```python
from build123d import *

# Parameters (mm, degrees)
F0_R     = 70
F0_W     = 10
F0_H     = 43.5
F0_W_2   = 43.5
F0_H_2   = 10
F0_R_2   = 4
F1_DEPTH = 5


with BuildPart() as f1:
    # F0 (on Top) → F1 (new body)
    with BuildSketch(Plane.XY):
        Circle(F0_R)
        with BuildLine():
            ThreePointArc((-50.419256, -41.023148), (-50.834826, -39.398712), (-49.867894, -38.028846))
            Line((-49.867894, -38.028846), (-28.320508, -25.588457))
            ThreePointArc((-28.320508, -25.588457), (-25.906295, -25.906295), (-25.588457, -28.320508))
            Line((-25.588457, -28.320508), (-38.028846, -49.867894))
            ThreePointArc((-38.028846, -49.867894), (-39.398712, -50.834826), (-41.023148, -50.419256))
            ThreePointArc((-41.023148, -50.419256), (-45.961941, -45.961941), (-50.419256, -41.023148))
        make_face(mode=Mode.SUBTRACT)
        Polygon((-6.669873, -21.552559), (-28.419873, -59.224664), (-37.080127, -54.224664), (-15.330127, -16.552559), align=None, mode=Mode.SUBTRACT)
        with BuildLine():
            ThreePointArc((-23.152782, -60.736716), (-24.324895, -59.537699), (-24.17244, -57.867894))
            Line((-24.17244, -57.867894), (-11.732051, -36.320508))
            ThreePointArc((-11.732051, -36.320508), (-9.482362, -35.388656), (-8, -37.320508))
            Line((-8, -37.320508), (-8, -62.201286))
            ThreePointArc((-8, -62.201286), (-8.702873, -63.723607), (-10.31746, -64.17593))
            ThreePointArc((-10.31746, -64.17593), (-16.823238, -62.785179), (-23.152782, -60.736716))
        make_face(mode=Mode.SUBTRACT)
        Polygon((-16.552559, -15.330127), (-54.224664, -37.080127), (-59.224664, -28.419873), (-21.552559, -6.669873), align=None, mode=Mode.SUBTRACT)
        with BuildLine():
            ThreePointArc((-64.17593, -10.31746), (-63.723607, -8.702873), (-62.201286, -8))
            Line((-62.201286, -8), (-37.320508, -8))
            ThreePointArc((-37.320508, -8), (-35.388656, -9.482362), (-36.320508, -11.732051))
            Line((-36.320508, -11.732051), (-57.867894, -24.17244))
            ThreePointArc((-57.867894, -24.17244), (-59.537699, -24.324895), (-60.736716, -23.152782))
            ThreePointArc((-60.736716, -23.152782), (-62.785179, -16.823238), (-64.17593, -10.31746))
        make_face(mode=Mode.SUBTRACT)
        with BuildLine():
            ThreePointArc((10.31746, -64.17593), (8.702873, -63.723607), (8, -62.201286))
            Line((8, -62.201286), (8, -37.320508))
            ThreePointArc((8, -37.320508), (9.482362, -35.388656), (11.732051, -36.320508))
            Line((11.732051, -36.320508), (24.17244, -57.867894))
            ThreePointArc((24.17244, -57.867894), (24.324895, -59.537699), (23.152782, -60.736716))
            ThreePointArc((23.152782, -60.736716), (16.823238, -62.785179), (10.31746, -64.17593))
        make_face(mode=Mode.SUBTRACT)
        with Locations((0, -43.75)):
            Rectangle(F0_W, F0_H, mode=Mode.SUBTRACT)
        Polygon((15.330127, -16.552559), (37.080127, -54.224664), (28.419873, -59.224664), (6.669873, -21.552559), align=None, mode=Mode.SUBTRACT)
        with BuildLine():
            ThreePointArc((41.023148, -50.419256), (39.398712, -50.834826), (38.028846, -49.867894))
            Line((38.028846, -49.867894), (25.588457, -28.320508))
            ThreePointArc((25.588457, -28.320508), (25.906295, -25.906295), (28.320508, -25.588457))
            Line((28.320508, -25.588457), (49.867894, -38.028846))
            ThreePointArc((49.867894, -38.028846), (50.834826, -39.398712), (50.419256, -41.023148))
            ThreePointArc((50.419256, -41.023148), (45.961941, -45.961941), (41.023148, -50.419256))
        make_face(mode=Mode.SUBTRACT)
        Polygon((21.552559, -6.669873), (59.224664, -28.419873), (54.224664, -37.080127), (16.552559, -15.330127), align=None, mode=Mode.SUBTRACT)
        with BuildLine():
            ThreePointArc((60.736716, -23.152782), (59.537699, -24.324895), (57.867894, -24.17244))
            Line((57.867894, -24.17244), (36.320508, -11.732051))
            ThreePointArc((36.320508, -11.732051), (35.388656, -9.482362), (37.320508, -8))
            Line((37.320508, -8), (62.201286, -8))
            ThreePointArc((62.201286, -8), (63.723607, -8.702873), (64.17593, -10.31746))
            ThreePointArc((64.17593, -10.31746), (62.785179, -16.823238), (60.736716, -23.152782))
        make_face(mode=Mode.SUBTRACT)
        with Locations((-43.75, 0)):
            Rectangle(F0_W_2, F0_H_2, mode=Mode.SUBTRACT)
        with BuildLine():
            ThreePointArc((-60.736716, 23.152782), (-59.537699, 24.324895), (-57.867894, 24.17244))
            Line((-57.867894, 24.17244), (-36.320508, 11.732051))
            ThreePointArc((-36.320508, 11.732051), (-35.388656, 9.482362), (-37.320508, 8))
            Line((-37.320508, 8), (-62.201286, 8))
            ThreePointArc((-62.201286, 8), (-63.723607, 8.702873), (-64.17593, 10.31746))
            ThreePointArc((-64.17593, 10.31746), (-62.785179, 16.823238), (-60.736716, 23.152782))
        make_face(mode=Mode.SUBTRACT)
        Polygon((-21.552559, 6.669873), (-59.224664, 28.419873), (-54.224664, 37.080127), (-16.552559, 15.330127), align=None, mode=Mode.SUBTRACT)
        with BuildLine():
            ThreePointArc((-41.023148, 50.419256), (-39.398712, 50.834826), (-38.028846, 49.867894))
            Line((-38.028846, 49.867894), (-25.588457, 28.320508))
            ThreePointArc((-25.588457, 28.320508), (-25.906295, 25.906295), (-28.320508, 25.588457))
            Line((-28.320508, 25.588457), (-49.867894, 38.028846))
            ThreePointArc((-49.867894, 38.028846), (-50.834826, 39.398712), (-50.419256, 41.023148))
            ThreePointArc((-50.419256, 41.023148), (-45.961941, 45.961941), (-41.023148, 50.419256))
        make_face(mode=Mode.SUBTRACT)
        Polygon((-15.330127, 16.552559), (-37.080127, 54.224664), (-28.419873, 59.224664), (-6.669873, 21.552559), align=None, mode=Mode.SUBTRACT)
        with BuildLine():
            Line((-11.732051, 36.320508), (-24.17244, 57.867894))
            ThreePointArc((-24.17244, 57.867894), (-24.324895, 59.537699), (-23.152782, 60.736716))
            ThreePointArc((-23.152782, 60.736716), (-16.823238, 62.785179), (-10.31746, 64.17593))
            ThreePointArc((-10.31746, 64.17593), (-8.702873, 63.723607), (-8, 62.201286))
            Line((-8, 62.201286), (-8, 37.320508))
            ThreePointArc((-8, 37.320508), (-9.482362, 35.388656), (-11.732051, 36.320508))
        make_face(mode=Mode.SUBTRACT)
        Circle(F0_R_2, mode=Mode.SUBTRACT)
        with Locations((43.75, 0)):
            Rectangle(F0_W_2, F0_H_2, mode=Mode.SUBTRACT)
        with BuildLine():
            ThreePointArc((64.17593, 10.31746), (63.723607, 8.702873), (62.201286, 8))
            Line((62.201286, 8), (37.320508, 8))
            ThreePointArc((37.320508, 8), (35.388656, 9.482362), (36.320508, 11.732051))
            Line((36.320508, 11.732051), (57.867894, 24.17244))
            ThreePointArc((57.867894, 24.17244), (59.537699, 24.324895), (60.736716, 23.152782))
            ThreePointArc((60.736716, 23.152782), (62.785179, 16.823238), (64.17593, 10.31746))
        make_face(mode=Mode.SUBTRACT)
        Polygon((16.552559, 15.330127), (54.224664, 37.080127), (59.224664, 28.419873), (21.552559, 6.669873), align=None, mode=Mode.SUBTRACT)
        with Locations((0, 43.75)):
            Rectangle(F0_W, F0_H, mode=Mode.SUBTRACT)
        with BuildLine():
            Line((8, 37.320508), (8, 62.201286))
            ThreePointArc((8, 62.201286), (8.702873, 63.723607), (10.31746, 64.17593))
            ThreePointArc((10.31746, 64.17593), (16.823238, 62.785179), (23.152782, 60.736716))
            ThreePointArc((23.152782, 60.736716), (24.324895, 59.537699), (24.17244, 57.867894))
            Line((24.17244, 57.867894), (11.732051, 36.320508))
            ThreePointArc((11.732051, 36.320508), (9.482362, 35.388656), (8, 37.320508))
        make_face(mode=Mode.SUBTRACT)
        Polygon((6.669873, 21.552559), (28.419873, 59.224664), (37.080127, 54.224664), (15.330127, 16.552559), align=None, mode=Mode.SUBTRACT)
        with BuildLine():
            Line((25.588457, 28.320508), (38.028846, 49.867894))
            ThreePointArc((38.028846, 49.867894), (39.398712, 50.834826), (41.023148, 50.419256))
            ThreePointArc((41.023148, 50.419256), (45.961941, 45.961941), (50.419256, 41.023148))
            ThreePointArc((50.419256, 41.023148), (50.834826, 39.398712), (49.867894, 38.028846))
            Line((49.867894, 38.028846), (28.320508, 25.588457))
            ThreePointArc((28.320508, 25.588457), (25.906295, 25.906295), (25.588457, 28.320508))
        make_face(mode=Mode.SUBTRACT)
    extrude(amount=F1_DEPTH)


solid = f1.part
```
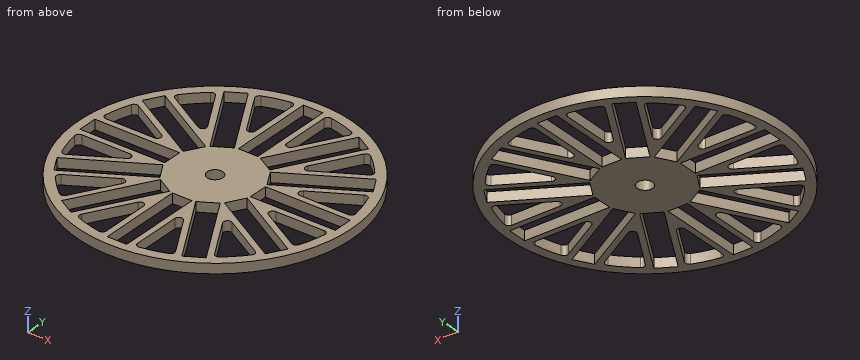
Input: part model. Units: mm. Frame: model coordinates. Give positions to 0.01 mm unless a question says otherwise; leave off trailing zeros. Order: outer loops, then holes, each group sorted by start corner. A loop starts at its lowest first (then second) coordinate and runs counter-clockwise, first axis right, second up. Notation, with made-up numbers: (55, 59.5) -> (71, 59.5) arc R24 ccw to (71, 88.5) -> close; hole circle Ø2 at (9.5, 52.25). An arc over 180 degrees is marked (long way). Write each question's results on one line, items separated by ' | '. Start each with the question number.
Item 1: Line query: line 1 (Y direction, x = 0, z = 2.4); line 2 (Y direction, x = 12.5, z = 4.05); line 3 (X direction, y = 56.5, z = 3.4). Output: solid intervals per line, ascending.
Item 2: Contact query for flat-ended pins moving along their axis: P1, Ø2, axis at y = 36.5, z = 2.5, coming from the -X side; P2, Ø3, axis at x = -10, y = -53, coming from the -Z side; P3, Ø2.5, axis at x = 47.5, z = 2, coming from the +Y side; P4, Ø1.5, axis at y = 49.5, z = 3, coming from the +X side. Output: stop coordinate, or through.
Item 3: Cut plane A-A on y = 0. Return the cut outline in (x, z), then the cut area to 3 significant figures.
Item 4: Cut plane C-C on y = -47.5. Give the number of separate pieces and of enclosed holes in the cut face, then the cut area to 3 significant figures.
Established:
1) line 1: -70 to -65.5, -22 to -4, 4 to 22, 65.5 to 70 | line 2: -68.87 to -63.79, -37.65 to -31.65, -18.19 to 18.19, 31.65 to 37.65, 63.79 to 68.87 | line 3: -41.32 to -33.14, -26.85 to -23.38, -8 to -5, 5 to 8, 23.38 to 26.85, 33.14 to 41.32
2) P1: x = -60.33 | P2: through | P3: y = 52.54 | P4: x = 50.23
3) outline: (-70, 0) -> (-65.5, 0) -> (-65.5, 5) -> (-70, 5) -> close; (-22, 0) -> (-4, 0) -> (-4, 5) -> (-22, 5) -> close; (4, 0) -> (22, 0) -> (22, 5) -> (4, 5) -> close; (65.5, 0) -> (70, 0) -> (70, 5) -> (65.5, 5) -> close | area: 225 mm^2
4) separate pieces: 8 | enclosed holes: 0 | area: 170 mm^2
